Input: part model. Units: mm. Frame: model coordinates. A direction names the side the tool comes from. Coordinates: 2 decimals unless noted, no trailing zeros. Loops run counter-clockwise (first coordinate to the right, second up) from the corner with the lowest first, then second, coordinate; pieces in that order, holes last. Notation, with made-up numbers: (71.25, 2) - (98.25, 2) arc R9 cw to (98.25, 12) - close; hole circle Ø5 at (47.5, 63.25). An arc over 180 degrees is marked (long way). Use a Markdown table: item, result. Add a question column.
1. Section query D-D on y = 8.2. State how many separate pieces and enclosed holes the cut face has, then the cut area to 3 significant figures.
2. Draft query along X for faces 5 (the face through (-7.3, 0, 8.7)), 6 (the face through (-24, -7.4, -13.5)), 7 (the face through (12.05, 14.07, 8.76)). Return one class per face: released by +X, released by -X, zero draft, split by the parting line, or undercut.
3. Contact query for flat-ended pins moving along their axis: P1, Ø4, axis at x = -19.5, y = 9, coming from the -Z side; P2, Ø6.5, axis at x = -20.5, y = 9.5, coming from the +Z side; P3, Ø1, axis at y = 8.5, z = -31, coming from the +X side; P4, Ø0.8, axis at x = -3, y = 1.5, coming from the -Z side. Output: stop coordinate, or through.
4. Ray query, L1, parallel to Z at x = -21, y = 4; L2, parallel to Z at x = -20.7, y = 8.2; L3, parallel to Y at x = -19.75, z = -41.3. Return the intervals inside material, ascending. Write a range as [from, to].
5. Section query B-B on y = -6.2. Return the cut outline in (x, z).
6. Access query for faces 1 (the face through (-21, 9, -32.809)), 2 (the face through (0, -1, 21.288)), 3 (the face through (-7.3, 2, 8.7)), 4 (the face through (10.864, -1, 18)). Directions: +Z, -Z, +X, -X, +Y, -Y. A direction counts if a zero-diameter tool reaches every point of the face in a straight line with its end or side. Return the directions, or none.
7. Section query A-A on z = -41.3. Return the cut outline in (x, y).
8. Section query C-C on z = 1.5. Return the cut outline in (x, y).
```python
from build123d import *

# Parameters (mm, degrees)
EXTRUDE_1_DEPTH      = 2
CUT_EXTRUDE_1_DEPTH  = 2
SKETCH_3_W           = 3
SKETCH_3_H           = 3
EXTRUDE_2_DEPTH      = 12
EXTRUDE_3_DEPTH      = 15
SKETCH_5_R           = 0.75
CUT_EXTRUDE_2_DEPTH  = 12
SKETCH_6_R           = 1.05
CUT_EXTRUDE_3_DEPTH  = 12
SKETCH_7_W           = 26
SKETCH_7_H           = 60
EXTRUDE_4_DEPTH      = 2
SKETCH_8_W           = 6
SKETCH_8_H           = 4.457179677
SKETCH_8_H_2         = 4.5
EXTRUDE_5_DEPTH      = 14.4
SKETCH_9_R           = 0.95
CUT_EXTRUDE_4_DEPTH  = 14.4
SKETCH_10_W          = 26
SKETCH_10_H          = 8
EXTRUDE_6_DEPTH      = 2
SKETCH_11_W          = 4.5
SKETCH_11_H          = 4.5
EXTRUDE_7_DEPTH      = 14.4
SKETCH_12_R          = 0.95
CUT_EXTRUDE_5_DEPTH  = 14.4
SKETCH_13_W          = 4.5
SKETCH_13_H          = 4.5
CUT_EXTRUDE_6_DEPTH  = 14.4
SKETCH_15_R          = 1.75
CUT_EXTRUDE_8_DEPTH  = 12
SKETCH_14_W          = 3
SKETCH_14_H          = 3
CUT_EXTRUDE_9_DEPTH  = 12
CUT_EXTRUDE_11_DEPTH = 10
CUT_EXTRUDE_13_DEPTH = 5
SKETCH_22_W          = 8.2
SKETCH_22_H          = 8.2
CUT_EXTRUDE_15_DEPTH = 1
SKETCH_23_W          = 10
SKETCH_23_H          = 49
CUT_EXTRUDE_16_DEPTH = 10
FILLET_4_R           = 1
SKETCH_24_W          = 19.2
SKETCH_24_H          = 5.2
CUT_EXTRUDE_17_DEPTH = 1
EXTRUDE_START        = -1
SKETCH_25_W          = 21.2
SKETCH_25_H          = 7.2
SKETCH_25_R          = 1.75
EXTRUDE_10_DEPTH     = 2
FILLET_5_R           = 1
CUT_EXTRUDE_18_DEPTH = 10
CUT_EXTRUDE_19_DEPTH = 10
FILLET_7_R           = 1
EXTRUDE_12_DEPTH     = 6
SKETCH_34_R          = 1
CUT_EXTRUDE_24_DEPTH = 10
FILLET_9_R           = 1
SKETCH_31_W          = 28.262434414
SKETCH_31_H          = 5.377761842
CUT_EXTRUDE_22_DEPTH = 10
SKETCH_32_R          = 1.7
CUT_EXTRUDE_23_DEPTH = 10


with BuildPart() as part:
    # 草图1 → 凸台-拉伸1 (new body)
    with BuildSketch(Plane(origin=(0, 0, 0), x_dir=(1, 0, 0), z_dir=(0, 1, 0))):
        with BuildLine():
            Line((5, 0), (31, 0))
            Line((31, 0), (31, -12.266105287))
            Line((31, -12.266105287), (17.561663747, -40))
            Line((17.561663747, -40), (-17.561663747, -40))
            Line((-17.561663747, -40), (-31, -12.266105287))
            Line((-31, -12.266105287), (-31, 0))
            Line((-31, 0), (-5, 0))
            Line((-5, 0), (-5, -5))
            ThreePointArc((-5, -5), (0, -10), (5, -5))
            Line((5, -5), (5, 0))
        make_face()
    extrude(amount=EXTRUDE_1_DEPTH)

    # 草图2 → 切除-拉伸1 (cut)
    with BuildSketch(Plane.XZ):
        Polygon((-31, 0), (-24.370648345, 19.60824232), (-13.01326486, 35.515995577), (-4.410164775, 40), (-17.561663747, 40), (-31, 12.266105287), align=None)
    cut_extrude_1 = extrude(amount=-CUT_EXTRUDE_1_DEPTH, mode=Mode.SUBTRACT)

    # 镜向1: 切除-拉伸1 across plane
    add(cut_extrude_1.mirror(Plane(origin=(0, 0, 0), x_dir=(0, 0, 1), z_dir=(1, 0, 0))), mode=Mode.SUBTRACT)

    # 草图3 → 凸台-拉伸2 (add)
    with BuildSketch(Plane(origin=(0, 2, 0), x_dir=(1, 0, 0), z_dir=(0, 1, 0))):
        with Locations((0.264476572, -30.687696452)):
            Rectangle(SKETCH_3_W, SKETCH_3_H)
    extrude(amount=EXTRUDE_2_DEPTH)

    # 草图4 → 凸台-拉伸3 (add)
    with BuildSketch(Plane(origin=(0, 2, 0), x_dir=(1, 0, 0), z_dir=(0, 1, 0))):
        Polygon((12.4652939, -10.808762302), (14.186023209, -8.35130617), (15.6199643, -6.303426059), (12.343356123, -4.009120313), (10.909415032, -6.057000424), (9.188685723, -8.514456557), (7.754744632, -10.562336668), (11.031352809, -12.856642413), align=None)
    extrude_3 = extrude(amount=EXTRUDE_3_DEPTH)

    # 草图5 → 切除-拉伸2 (cut)
    with BuildSketch(Plane.ZY.offset(1.235523428)):
        with Locations((30.687696452, 11.5)):
            Circle(SKETCH_5_R)
        with Locations((30.687696452, 4.5)):
            Circle(SKETCH_5_R)
    extrude(amount=-CUT_EXTRUDE_2_DEPTH, mode=Mode.SUBTRACT)

    # 草图6 → 切除-拉伸3 (cut)
    with BuildSketch(Plane(origin=(25.938855932, 0, 23.294988476), x_dir=(0.8191520442889928, 0, 0.5735764363510446), z_dir=(-0.5735764363510446, 0, 0.8191520442889928))):
        with Locations((-20.198700994, 15)):
            Circle(SKETCH_6_R)
        with Locations((-20.198700994, 6)):
            Circle(SKETCH_6_R)
    cut_extrude_3 = extrude(amount=-CUT_EXTRUDE_3_DEPTH, mode=Mode.SUBTRACT)

    # 镜向2: 凸台-拉伸3, 切除-拉伸3 across plane
    add(extrude_3.mirror(Plane(origin=(0, 0, 0), x_dir=(0, 0, 1), z_dir=(1, 0, 0))))
    add(cut_extrude_3.mirror(Plane(origin=(0, 0, 0), x_dir=(0, 0, 1), z_dir=(1, 0, 0))), mode=Mode.SUBTRACT)

    # 草图7 → 凸台-拉伸4 (add)
    with BuildSketch(Plane(origin=(0, 2, 0), x_dir=(1, 0, 0), z_dir=(0, 1, 0))):
        with Locations((-18, 30)):
            Rectangle(SKETCH_7_W, SKETCH_7_H)
        with Locations((18, 30)):
            Rectangle(SKETCH_7_W, SKETCH_7_H)
    extrude(amount=-EXTRUDE_4_DEPTH)

    # 草图8 → 凸台-拉伸5 (add)
    with BuildSketch(Plane(origin=(0, 2, 0), x_dir=(1, 0, 0), z_dir=(0, 1, 0))):
        with Locations((20.92336727, 3.180021452)):
            Rectangle(SKETCH_8_W, SKETCH_8_H)
        with Locations((20.92336727, 30.55861129)):
            Rectangle(SKETCH_8_W, SKETCH_8_H_2)
    extrude_5 = extrude(amount=EXTRUDE_5_DEPTH)

    # 草图9 → 切除-拉伸4 (cut)
    with BuildSketch(Plane(origin=(31, 0, 0), x_dir=(0, 0, -1), z_dir=(1, 0, 0))):
        with Locations((3.00861129, 8.2)):
            Circle(SKETCH_9_R)
        with Locations((30.70861129, 8.2)):
            Circle(SKETCH_9_R)
    cut_extrude_4 = extrude(amount=-CUT_EXTRUDE_4_DEPTH, mode=Mode.SUBTRACT)

    # 镜向3: 凸台-拉伸5, 切除-拉伸4 across plane
    add(extrude_5.mirror(Plane(origin=(0, 0, 0), x_dir=(0, 0, 1), z_dir=(1, 0, 0))))
    add(cut_extrude_4.mirror(Plane(origin=(0, 0, 0), x_dir=(0, 0, 1), z_dir=(1, 0, 0))), mode=Mode.SUBTRACT)

    # 草图10 → 凸台-拉伸6 (add)
    with BuildSketch(Plane(origin=(0, 2, 0), x_dir=(1, 0, 0), z_dir=(0, 1, 0))):
        with Locations((-18, 64)):
            Rectangle(SKETCH_10_W, SKETCH_10_H)
        Polygon((5, 60), (5, 68), (30.798641436, 68), (31, 60), align=None)
    extrude(amount=-EXTRUDE_6_DEPTH)

    # 草图11 → 凸台-拉伸7 (add)
    with BuildSketch(Plane(origin=(0, 2, 0), x_dir=(1, 0, 0), z_dir=(0, 1, 0))):
        with Locations((18.529999999, 37.05861129)):
            Rectangle(SKETCH_11_W, SKETCH_11_H)
        with Locations((18.529999999, 64.45861129)):
            Rectangle(SKETCH_11_W, SKETCH_11_H)
    extrude(amount=EXTRUDE_7_DEPTH)

    # 草图12 → 切除-拉伸5 (cut)
    with BuildSketch(Plane.ZY.offset(-16.279999999)):
        with Locations((-36.90861129, 8.2)):
            Circle(SKETCH_12_R)
        with Locations((-64.60861129, 8.2)):
            Circle(SKETCH_12_R)
    extrude(amount=-CUT_EXTRUDE_5_DEPTH, mode=Mode.SUBTRACT)

    # 草图13 → 切除-拉伸6 (cut)
    with BuildSketch(Plane(origin=(0, 16.4, 0), x_dir=(1, 0, 0), z_dir=(0, 1, 0))):
        with Locations((18.529999999, 37.05861129)):
            Rectangle(SKETCH_13_W, SKETCH_13_H)
        with Locations((18.529999999, 64.45861129)):
            Rectangle(SKETCH_13_W, SKETCH_13_H)
    extrude(amount=-CUT_EXTRUDE_6_DEPTH, mode=Mode.SUBTRACT)

    # 草图15 → 切除-拉伸8 (cut)
    with BuildSketch(Plane(origin=(0, 2, 0), x_dir=(1, 0, 0), z_dir=(0, 1, 0))):
        with Locations(Location((-6.235523428, -17.687696452, 0), (0, 0, 270))):
            Circle(SKETCH_15_R)
        with Locations(Location((6.764476572, -17.687696452, 0), (0, 0, 270))):
            Circle(SKETCH_15_R)
    extrude(amount=-CUT_EXTRUDE_8_DEPTH, mode=Mode.SUBTRACT)

    # 草图14 → 切除-拉伸9 (cut)
    with BuildSketch(Plane(origin=(0, 14, 0), x_dir=(1, 0, 0), z_dir=(0, 1, 0))):
        with Locations((0.264476572, -30.687696452)):
            Rectangle(SKETCH_14_W, SKETCH_14_H)
    extrude(amount=-CUT_EXTRUDE_9_DEPTH, mode=Mode.SUBTRACT)

    # 草图17 → 切除-拉伸11 (cut)
    with BuildSketch(Plane.XZ):
        Polygon((-20.533375452, -44), (-31, -44), (-37, -44), (-37, -68), (-31, -68), (30.798641436, -68), (38, -68), (38, -44), (31, -44), align=None)
    extrude(amount=-CUT_EXTRUDE_11_DEPTH, mode=Mode.SUBTRACT)

    # 草图20 → 切除-拉伸13 (cut, symmetric)
    with BuildSketch(Plane.XZ):
        with BuildLine():
            Line((5, -44), (8, -44))
            Line((8, -44), (8, 5))
            ThreePointArc((8, 5), (0, 13), (-8, 5))
            Line((-8, 5), (-8, -44))
            Line((-8, -44), (5, -44))
        make_face()
    extrude(amount=CUT_EXTRUDE_13_DEPTH, both=True, mode=Mode.SUBTRACT)

    # 草图22 → 切除-拉伸15 (cut)
    with BuildSketch(Plane(origin=(0, 2, 0), x_dir=(1, 0, 0), z_dir=(0, 1, 0))):
        with Locations((24.1, -4.499009955)):
            Rectangle(SKETCH_22_W, SKETCH_22_H)
        with Locations((-24.1, -4.499009955)):
            Rectangle(SKETCH_22_W, SKETCH_22_H)
    extrude(amount=-CUT_EXTRUDE_15_DEPTH, mode=Mode.SUBTRACT)

    # 草图23 → 切除-拉伸16 (cut)
    with BuildSketch(Plane(origin=(0, 2, 0), x_dir=(1, 0, 0), z_dir=(0, 1, 0))):
        with Locations((13, 19.5)):
            Rectangle(SKETCH_23_W, SKETCH_23_H)
    cut_extrude_16 = extrude(amount=-CUT_EXTRUDE_16_DEPTH, mode=Mode.SUBTRACT)

    # 镜向6: 切除-拉伸16 across plane
    add(cut_extrude_16.mirror(Plane(origin=(0, 0, 0), x_dir=(0, 0, 1), z_dir=(1, 0, 0))), mode=Mode.SUBTRACT)

    # 圆角4
    fillet_4_edges = [part.edges().sort_by_distance(p)[0] for p in [
        (-8, 1, 5),
        (8, 1, 5),
        (18, 1, 5),
        (-18, 1, 5),
    ]]
    fillet(fillet_4_edges, radius=FILLET_4_R)

    # 草图24 → 切除-拉伸17 (cut)
    with BuildSketch(Plane(origin=(0, 2, 0), x_dir=(1, 0, 0), z_dir=(0, 1, 0))):
        with Locations((0.264476572, -17.687625884)):
            Rectangle(SKETCH_24_W, SKETCH_24_H)
    extrude(amount=-CUT_EXTRUDE_17_DEPTH, mode=Mode.SUBTRACT)

    # 草图25 → 凸台-拉伸10 (add)
    with BuildSketch(Plane(origin=(0, 1, 0), x_dir=(1, 0, 0), z_dir=(0, 1, 0)).offset(EXTRUDE_START)):
        with Locations((0.264476572, -17.687625884)):
            Rectangle(SKETCH_25_W, SKETCH_25_H)
        with Locations(Location((-6.235523428, -17.687696452, 0), (0, 0, 270))):
            Circle(SKETCH_25_R, mode=Mode.SUBTRACT)
        with Locations(Location((6.764476572, -17.687696452, 0), (0, 0, 270))):
            Circle(SKETCH_25_R, mode=Mode.SUBTRACT)
    extrude(amount=-EXTRUDE_10_DEPTH)

    # 圆角5
    fillet_5_edges = [part.edges().sort_by_distance(p)[0] for p in [
        (10.864476572, -1, 14.087625884),
        (10.864476572, -1, 21.287625884),
        (-10.335523428, -1, 21.287625884),
        (-10.335523428, -1, 14.087625884),
    ]]
    fillet(fillet_5_edges, radius=FILLET_5_R)

    # 草图26 → 切除-拉伸18 (cut)
    with BuildSketch(Plane(origin=(0, 2, 0), x_dir=(1, 0, 0), z_dir=(0, 1, 0))):
        with BuildLine():
            Line((-35.006467671, 0), (-35.006467671, -42.039018824))
            Line((-35.006467671, -42.039018824), (35.006467671, -42.039018824))
            Line((35.006467671, -42.039018824), (35.006467671, 0))
            ThreePointArc((35.006467671, 0), (0, -35.006467671), (-35.006467671, 0))
        make_face()
    extrude(amount=-CUT_EXTRUDE_18_DEPTH, mode=Mode.SUBTRACT)

    # 草图27 → 切除-拉伸19 (cut)
    with BuildSketch(Plane(origin=(0, 2, 0), x_dir=(1, 0, 0), z_dir=(0, 1, 0))):
        Polygon((-27.379819186, -10.707741319), (-14.131217207, -29.628705829), (-14.131217207, -32.027511284), (-27.379819186, -32.027511284), align=None)
    cut_extrude_19 = extrude(amount=-CUT_EXTRUDE_19_DEPTH, mode=Mode.SUBTRACT)

    # 镜向4: 切除-拉伸19 across plane
    add(cut_extrude_19.mirror(Plane(origin=(0, 0, 0), x_dir=(0, 0, 1), z_dir=(1, 0, 0))), mode=Mode.SUBTRACT)

    # 圆角7
    fillet_7_edges = [part.edges().sort_by_distance(p)[0] for p in [
        (23.92336727, 9.2, -5.40861129),
        (23.92336727, 9.2, -28.30861129),
        (-23.92336727, 9.2, -5.40861129),
        (-23.92336727, 9.2, -28.30861129),
    ]]
    fillet(fillet_7_edges, radius=FILLET_7_R)

    # 草图33 → 凸台-拉伸12 (add)
    with BuildSketch(Plane.ZY.offset(24)):
        Polygon((-44, 0), (-44, -15), (-39, -15), (-39, 0), (-39, 2), (-44, 2), align=None)
        Polygon((-16, 0), (-16, -15), (-11, -15), (-11, 0), (-11, 2), (-16, 2), align=None)
    extrude(amount=-EXTRUDE_12_DEPTH)

    # 草图34 → 切除-拉伸24 (cut)
    with BuildSketch(Plane(origin=(-18, 0, 0), x_dir=(0, 0, -1), z_dir=(1, 0, 0))):
        with Locations((13.6, -6.2)):
            Circle(SKETCH_34_R)
        with Locations((41.3, -6.2)):
            Circle(SKETCH_34_R)
    extrude(amount=-CUT_EXTRUDE_24_DEPTH, mode=Mode.SUBTRACT)

    # 圆角9
    fillet_9_edges = [part.edges().sort_by_distance(p)[0] for p in [
        (-18, -7.5, -39),
        (-18, -7.5, -16),
    ]]
    fillet(fillet_9_edges, radius=FILLET_9_R)

    # 草图31 → 切除-拉伸22 (cut)
    with BuildSketch(Plane(origin=(0, 2, 0), x_dir=(1, 0, 0), z_dir=(0, 1, 0))):
        with Locations((0, -32.31758675)):
            Rectangle(SKETCH_31_W, SKETCH_31_H)
    extrude(amount=-CUT_EXTRUDE_22_DEPTH, mode=Mode.SUBTRACT)

    # 草图32 → 切除-拉伸23 (cut)
    with BuildSketch(Plane(origin=(0, 1, 0), x_dir=(1, 0, 0), z_dir=(0, 1, 0))):
        with Locations(Location((-24.1, -4.499009955, 0), (0, 0, 270))):
            Circle(SKETCH_32_R)
        with Locations(Location((24.1, -4.499009955, 0), (0, 0, 270))):
            Circle(SKETCH_32_R)
    extrude(amount=-CUT_EXTRUDE_23_DEPTH, mode=Mode.SUBTRACT)


solid = part.part
```
Resolved:
| question | item | result |
|---|---|---|
| 1 | separate pieces | 10 |
| 1 | enclosed holes | 0 |
| 1 | area | 125 mm² |
| 2 | face 5 | zero draft |
| 2 | face 6 | released by -X |
| 2 | face 7 | undercut |
| 3 | P1 | z = -32.81 |
| 3 | P2 | z = -0.95 |
| 3 | P3 | through |
| 3 | P4 | z = 12.24 |
| 4 | L1 | [-32.81, -28.31], [-5.41, -0.95] |
| 4 | L2 | [-32.81, -31.66], [-29.76, -28.31], [-5.41, -3.96], [-2.06, -0.95] |
| 4 | L3 | [-15, -7.2], [-5.2, 2] |
| 5 | outline | (-24, -44) - (-18, -44) - (-18, -42.3) - (-24, -42.3) - close; (-24, -40.3) - (-18, -40.3) - (-18, -40) arc R1 ccw to (-19, -39) - (-24, -39) - close; (-24, -16) - (-19, -16) arc R1 ccw to (-18, -15) - (-18, -14.6) - (-24, -14.6) - close; (-24, -12.6) - (-18, -12.6) - (-18, -11) - (-24, -11) - close |
| 6 | face 1 | -Z, +X, -X, +Y |
| 6 | face 2 | +Z, +X, -X, -Y |
| 6 | face 3 | +Y |
| 6 | face 4 | +Z, -Z, +X, -Y |
| 7 | outline | (-31, 0) - (-24, 0) - (-24, -5.2) - (-18, -5.2) - (-18, 2) - (-31, 2) - close; (-24, -15) - (-18, -15) - (-18, -7.2) - (-24, -7.2) - close; (18, 0) - (31, 0) - (31, 2) - (18, 2) - close |
| 8 | outline | (-30.49, 0) - (-18, 0) - (-18, 2) - (-20, 2) - (-20, 1) - (-28.2, 1) - (-28.2, 2) - (-30.49, 2) - close; (18, 0) - (30.49, 0) - (30.49, 2) - (28.2, 2) - (28.2, 1) - (20, 1) - (20, 2) - (18, 2) - close |
